Build history of the part. All positions in model axes, mm. A direction names the side the tool comes from. Give positions to 0.01 mm unless a question says otherwise; leave off trailing zeros. Order: outer loops, then holes, each group sorted by start corner. A loop starts at its lowest first (then second) coordinate and runs counter-clockwise, first axis right, second up. Notation, with made-up numbers: (74.25, -22) - (121.25, -22) arc R24 ccw to (121.25, -10) - close; hole circle Ø11 at (58.25, -27). An arc over 180 degrees is marked (long way). Use a Markdown table: item, result.
from build123d import *

# Parameters (mm, degrees)
F1_DEPTH = 20


with BuildPart() as f1:
    # F0 (on Right) → F1 (new body)
    with BuildSketch(Plane.YZ):
        with BuildLine():
            Line((18, -2), (17.88854382, -2))
            ThreePointArc((17.88854382, -2), (16.9075605646, -6.1753053167), (14.9666295471, -10))
            Line((14.9666295471, -10), (18, -10))
            Line((18, -10), (18, -2))
        make_face()
        with BuildLine():
            Line((18, -10), (14.9666295471, -10))
            ThreePointArc((14.9666295471, -10), (8.4852813742, -15.8745078664), (0, -18))
            Line((0, -18), (14.3178210633, -18))
            ThreePointArc((14.3178210633, -18), (16.2634559673, -16.2634559673), (18, -14.3178210633))
            Line((18, -14.3178210633), (18, -10))
        make_face()
        with BuildLine():
            Line((-14.3178210633, -18), (0, -18))
            ThreePointArc((0, -18), (-8.4852813742, -15.8745078664), (-14.9666295471, -10))
            Line((-14.9666295471, -10), (-18, -10))
            Line((-18, -10), (-18, -14.3178210633))
            ThreePointArc((-18, -14.3178210633), (-16.2634559673, -16.2634559673), (-14.3178210633, -18))
        make_face()
        with BuildLine():
            Line((14.3178210633, -18), (0, -18))
            Line((0, -18), (-14.3178210633, -18))
            ThreePointArc((-14.3178210633, -18), (0, -23), (14.3178210633, -18))
        make_face()
        with BuildLine():
            ThreePointArc((-14.9666295471, -10), (-16.9075605646, -6.1753053167), (-17.88854382, -2))
            Line((-17.88854382, -2), (-18, -2))
            Line((-18, -2), (-18, -10))
            Line((-18, -10), (-14.9666295471, -10))
        make_face()
        with BuildLine():
            Line((18, -18), (14.3178210633, -18))
            ThreePointArc((14.3178210633, -18), (0, -23), (-14.3178210633, -18))
            Line((-14.3178210633, -18), (-17, -18))
            Line((-17, -18), (-18, -18))
            Line((-18, -18), (-18, -19))
            Line((-18, -19), (-30.5, -19))
            Line((-30.5, -19), (-30.5, -28))
            Line((-30.5, -28), (30.5, -28))
            Line((30.5, -28), (30.5, -19))
            Line((30.5, -19), (18, -19))
            Line((18, -19), (18, -18))
        make_face()
        with BuildLine():
            ThreePointArc((18, -14.3178210633), (16.2634559673, -16.2634559673), (14.3178210633, -18))
            Line((14.3178210633, -18), (18, -18))
            Line((18, -18), (18, -14.3178210633))
        make_face()
        with BuildLine():
            Line((-17, -18), (-14.3178210633, -18))
            ThreePointArc((-14.3178210633, -18), (-16.2634559673, -16.2634559673), (-18, -14.3178210633))
            Line((-18, -14.3178210633), (-18, -18))
            Line((-18, -18), (-17, -18))
        make_face()
    extrude(amount=F1_DEPTH)


solid = f1.part
1) Slice it at A-A (z = -6). Write the cut outline in (x, y), and give its area (3 significant figures).
Computed:
| item | result |
|---|---|
| outline | (0, -18) - (20, -18) - (20, -16.97) - (0, -16.97) - close; (0, 16.97) - (20, 16.97) - (20, 18) - (0, 18) - close |
| area | 41.2 mm² |
2) Slice it at D-D (z = -15.75). Write the cut outline in (x, y), and give its area (3 significant figures).
Computed:
| item | result |
|---|---|
| outline | (0, -18) - (20, -18) - (20, -8.71) - (0, -8.71) - close; (0, 8.71) - (20, 8.71) - (20, 18) - (0, 18) - close |
| area | 371 mm² |
3) Two-plate mould, pull along X, no slides. Class faces 1 (the flat face through (20, 0, -21)), 2 (the flat face through (0, 0, -21)), 3 (the flat face through (10, -30.5, -23)): +X half, -X half, draft (parallel to the pull), parting line (faces both ways), or undercut.
Computed:
| item | result |
|---|---|
| face 1 | +X half |
| face 2 | -X half |
| face 3 | draft |
4) Wall check: line 1 (Z direction, x = 1.5, y = -26); line 2 (Y direction, x = 5.5, z = -3); line 3 (Y direction, x = 16.5, z = -4.5). Give the ranges that are in metal, low to high. Write a range as from..to.
Computed:
| item | result |
|---|---|
| line 1 | z = -28..-19 |
| line 2 | y = -18..-17.75, 17.75..18 |
| line 3 | y = -18..-17.43, 17.43..18 |
5) Pin check, flat tips, straight feed: P1, Ø5, axis at x = 8, z = -13.5, coming from the +Y side; P2, Ø6, axis at x = 10.5, y = -26.5, coming from the +Z side; P3, Ø10, axis at x = 7, y = -3.5, coming from the +Z side. Stop position of each tip, or through.
Computed:
| item | result |
|---|---|
| P1 | stops at y = 18 |
| P2 | stops at z = -19 |
| P3 | stops at z = -15.87 |
6) Slice it at C-C (y = 22). Write the cut outline in (x, z), and give its area (3 significant figures).
Computed:
| item | result |
|---|---|
| outline | (0, -28) - (20, -28) - (20, -19) - (0, -19) - close |
| area | 180 mm² |
7) Tool access for faces 4 (the flat face through (10, 30.5, -24)), 5 (the flat face through (10, 18, -11)), 6 (the flat face through (10, -18, -10)): list every direction of +Z, -Z, +X, -X, +Y, -Y with a clear straight run to the whole face (end or side of a thin tool).
Computed:
| item | result |
|---|---|
| face 4 | +Z, -Z, +X, -X, +Y |
| face 5 | +Z, +X, -X, +Y |
| face 6 | +Z, +X, -X, -Y |
8) Slice it at B-B (x = 15.25). Write the cut outline in (y, z), and give its area (3 significant figures).
Computed:
| item | result |
|---|---|
| outline | (-30.5, -28) - (30.5, -28) - (30.5, -19) - (18, -19) - (18, -2) - (17.89, -2) arc R18 cw to (-17.89, -2) - (-18, -2) - (-18, -19) - (-30.5, -19) - close |
| area | 724 mm² |
